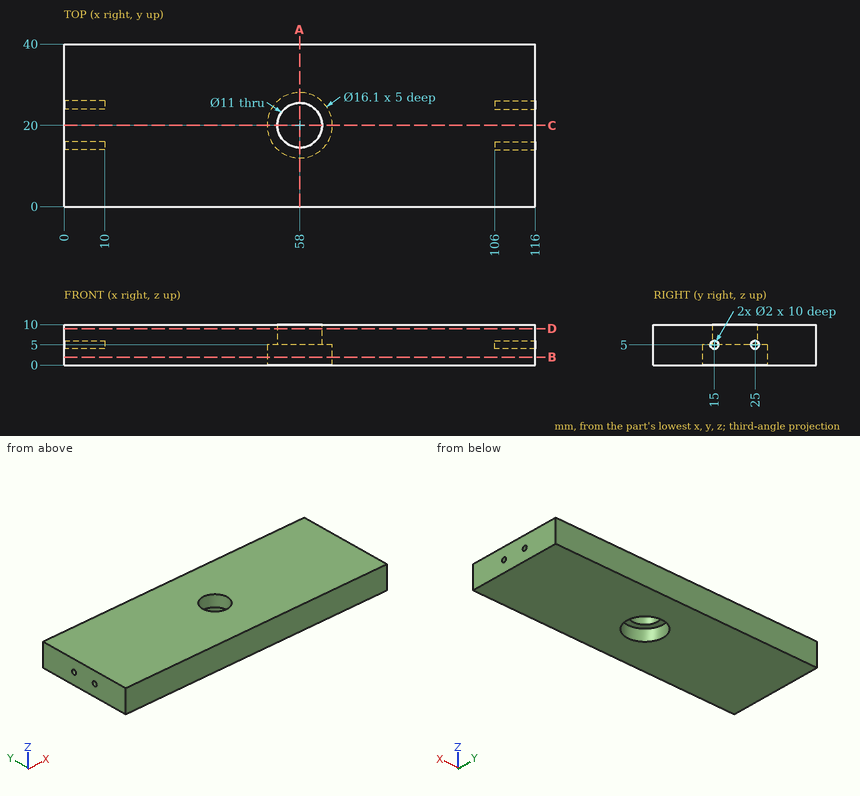
Can you work these out from the drawing? Everything is in mm from the part's minimum corner. Coordinates: 2 decimals unless noted, no trailing zeros. Loops run counter-clockwise (first coordinate to the right, second up) from the corner with the lowest first, then second, coordinate; pieces in that order, holes last. Notation, with made-up numbers: (88, -3.75) - (132, -3.75) arc R26 cw to (132, 23.25) - close; hole circle Ø1 at (-16, 82). An arc over 180 degrees is marked (long way). Put each result on its own line as item: value. Start each with the question number.
Item 1: Suppose I cut it at D-D (z = 9). Please give me the cut outline in (x, y), and give its area (3 significant figures).
Item 2: If I drill on line 1 along Y through (x, z) = (2.5, 5); line 2 along Y through (x, z) = (63, 9.75); line 3 along X through (y, z) = (24, 8), over which ranges is the centre line in solid material (lowest first)?
Item 3: For pin 1 (1.6 mm diameter, centred on y = 25, z = 5, fed in from -X), with a flat end and sliding along its axis, tell me the tip position at first contact or that it passes through.
Item 4: Suppose I cut it at B-B (z = 2). Please give me the cut outline in (x, y), and give its area (3 significant figures).
Item 5: Suppose I cut it at C-C (y = 20). Please give me the cut outline in (x, z), and give its area (3 significant figures).
Item 6: Suppose I cut it at A-A (x = 58). Please give me the cut outline in (y, z), and give its area (4 significant figures).
Here are the results:
1. outline: (0, 0) - (116, 0) - (116, 40) - (0, 40) - close; hole circle Ø11 at (58, 20)
1. area: 4,540 mm²
2. line 1: 0 to 14, 16 to 24, 26 to 40
2. line 2: 0 to 17.71, 22.29 to 40
2. line 3: 0 to 54.23, 61.77 to 116
3. pin 1: x = 10
4. outline: (0, 0) - (116, 0) - (116, 40) - (0, 40) - close; hole circle Ø16.1 at (58, 20)
4. area: 4,440 mm²
5. outline: (0, 0) - (49.95, 0) - (49.95, 5) - (52.5, 5) - (52.5, 10) - (0, 10) - close; (63.5, 5) - (66.05, 5) - (66.05, 0) - (116, 0) - (116, 10) - (63.5, 10) - close
5. area: 1,020 mm²
6. outline: (0, 0) - (11.95, 0) - (11.95, 5) - (14.5, 5) - (14.5, 10) - (0, 10) - close; (25.5, 5) - (28.05, 5) - (28.05, 0) - (40, 0) - (40, 10) - (25.5, 10) - close
6. area: 264.5 mm²
